Source: CAD feature listing. Evaluate the final solid. Frame: model axes, mm. Coordinates: 2 decimals unless noted, no trailing zeros. Write each loop counter-clockwise with the first axis right and the second up, starting at its lowest first coordinate (ties: lowest second). Pieces come first, ordered by that corner, then holes. Notation, with made-up numbers: M -18,76 L -2,76 A27 cw -2,105 Z; hole C 39,-38.75 d1. An arc over 180 degrees is marked long. Write item = value, one per line. Start each with the question number.
1. Pin query (flat end, axial travel): pin 1 Ø1.2 at (x, y) = (0, 0) entering from -Z. Return the tip coordinate at first contact, or that it passes through.
2. Section query B-B (y = 60). Output: boundary loops of the cut face in (x, z) (3 decimals).
3. Section query A-A (z = 1.95). Give the number of separate pieces and of enclosed holes in the cut face, then the cut area to 3 significant figures.
4. Line query: line 1 along Y through (x, z) = (0, 2.55); line 2 along X through (y, z) = (86, 1.95); line 3 along X through (y, z) = (56, 2.65). Output: solid intervals per line, ascending.
Autodesk Fusion 360 part; units mm, degrees
sketch "Sketch1" plane through (0, 0, 0) normal (0, 0, 1) x (1, 0, 0)
  line L0 (99, 4.8) -> (99, -4.8)
  line L1 (-99, -4.8) -> (-99, 4.8)
  line L2 (-99, 9) -> (99, -9) construction
  line L3 (99, 9) -> (-99, -9) construction
  line L4 (6, 99) -> (-4.8, 99)
  line L5 (-4.8, -99) -> (4.8, -99)
  line L6 (9, 99) -> (-9, -99) construction
  line L7 (-9, 99) -> (9, -99) construction
  line L8 (-29, -9) -> (-94.8, -9)
  line L9 (94.8, -9) -> (29, -9)
  line L10 (0.8182, -9) -> (-0.8182, -9)
  line L11 (29, 9) -> (94.8, 9)
  line L12 (-94.8, 9) -> (-31.5, 9)
  line L13 (-0.8182, 9) -> (0.8182, 9)
  line L14 (-9, 94.8) -> (-9, 31.5)
  line L15 (-9, 0.8182) -> (-9, -0.8182)
  line L16 (-9, -29) -> (-9, -94.8)
  line L17 (9, -94.8) -> (9, -29)
  line L18 (9, 29) -> (9, 96)
  arc A0 (9, 29) -> (29, 9) centre (29, 29) ccw
  arc A1 (29, -9) -> (9, -29) centre (29, -29) ccw
  arc A2 (-9, -29) -> (-29, -9) centre (-29, -29) ccw
  arc A3 (-31.5, 9) -> (-9, 31.5) centre (-31.5, 31.5) ccw
  arc A4 (9, 96) -> (6, 99) centre (6, 96) ccw
  arc A5 (-4.8, 99) -> (-9, 94.8) centre (-4.8, 94.8) ccw
  arc A6 (-94.8, 9) -> (-99, 4.8) centre (-94.8, 4.8) ccw
  arc A7 (-99, -4.8) -> (-94.8, -9) centre (-94.8, -4.8) ccw
  arc A8 (99, 4.8) -> (94.8, 9) centre (94.8, 4.8) ccw
  arc A9 (94.8, -9) -> (99, -4.8) centre (94.8, -4.8) ccw
  arc A10 (-9, -94.8) -> (-4.8, -99) centre (-4.8, -94.8) ccw
  arc A11 (4.8, -99) -> (9, -94.8) centre (4.8, -94.8) ccw
  circle A12 centre (-86, 0) radius 1
  circle A13 centre (-31, 0) radius 1
  circle A14 centre (86, 0) radius 1
  circle A15 centre (31, 0) radius 1
  circle A16 centre (0, -86) radius 1
  circle A17 centre (0, -31) radius 1
  circle A18 centre (0, 86) radius 1
  circle A19 centre (0, 31) radius 1
  circle A20 centre (0, 0) radius 1
  dimension "d1" = 198
  dimension "d2" = 18
  dimension "d5" = 18
  dimension "d6" = 198
  dimension "d9" = 20
  dimension "d10" = 22.5
  dimension "d11" = 3
  dimension "d12" = 4.2
  dimension "d15" = 2
  dimension "d16" = 2
  dimension "d17" = 13
  dimension "d18" = 2
  dimension "d19" = 13
  dimension "d20" = 2
  dimension "d21" = 2
  dimension "d22" = 13
  dimension "d23" = 2
  dimension "d24" = 2
  dimension "d25" = 13
  dimension "d26" = 68
  dimension "d27" = 68
  dimension "d28" = 68
  dimension "d29" = 68
  dimension "d30" = 2
extrude "Extrude1" add sketch "Sketch1" along normal blind 3.175
equation "d1 = totalArmLenght"
equation "d2 = armWidth"
equation "totalArmLenght = 198 mm"
equation "armWidth = 18 mm"
equation "d5 = armWidth"
equation "d6 = totalArmLenght"
equation "tipBend = 13 mm"
equation "bottomBend = 68 mm"
equation "d17 = tipBend"
equation "d19 = tipBend"
equation "d22 = tipBend"
equation "d25 = tipBend"
equation "d26 = bottomBend"
equation "d27 = bottomBend"
equation "d28 = bottomBend"
equation "d29 = bottomBend"
Results are:
q1.pin_1 = through
q2.outline = M -9,0 L 9,0 L 9,3.175 L -9,3.175 Z
q3.separate_pieces = 1
q3.enclosed_holes = 9
q3.area = 7,110 mm^2
q4.line_1 = -99 to -87, -85 to -32, -30 to -1, 1 to 30, 32 to 85, 87 to 99
q4.line_2 = -9 to -1, 1 to 9
q4.line_3 = -9 to 9
